```python
from build123d import *

# Parameters (mm, degrees)
CROQUIS1_R              = 2
SALIENTE_EXTRUIR2_DEPTH = 5
CHAFL_N1_SIZE           = 2
CHAFL_N1_SIZE2          = 3.464101615
CROQUIS3_R              = 4
CROQUIS3_R_2            = 1.5
SALIENTE_EXTRUIR3_DEPTH = 5
CROQUIS4_W              = 5
CROQUIS4_H              = 40
SALIENTE_EXTRUIR4_DEPTH = 5
REDONDEO1_R             = 3


with BuildPart() as part:
    # Croquis1 → Saliente-Extruir2 (new body)
    with BuildSketch(Plane(origin=(0, 0, 0), x_dir=(1, 0, 0), z_dir=(0, 1, 0))):
        Polygon((-50, 45), (-50, -45), (50, -45), (50, 45), (15, 45), (15, 30), (-15, 30), (-15, 45), align=None)
        with Locations(Location((-36, -36.5, 0), (0, 0, 270))):
            Circle(CROQUIS1_R, mode=Mode.SUBTRACT)
        with Locations(Location((-36, 36.5, 0), (0, 0, 270))):
            Circle(CROQUIS1_R, mode=Mode.SUBTRACT)
        with Locations(Location((36, 36.5, 0), (0, 0, 270))):
            Circle(CROQUIS1_R, mode=Mode.SUBTRACT)
        with Locations(Location((36, -36.5, 0), (0, 0, 270))):
            Circle(CROQUIS1_R, mode=Mode.SUBTRACT)
    extrude(amount=SALIENTE_EXTRUIR2_DEPTH)

    # Chaflán1
    chafl_n1_edges = [part.edges().sort_by_distance(p)[0] for p in [
        (-36, 5, 34.5),
        (-36, 5, -38.5),
        (36, 5, -38.5),
        (36, 5, 34.5),
    ]]
    chafl_n1_side = [part.faces().sort_by_distance(p)[0] for p in [
        (0, 5, 1.985356127),
    ]]
    chamfer(chafl_n1_edges, length=CHAFL_N1_SIZE, length2=CHAFL_N1_SIZE2, reference=chafl_n1_side[0])

    # Croquis3 → Saliente-Extruir3 (add)
    # profile 1 of 4: a face of its own
    with BuildSketch(Plane(origin=(0, 5, 0), x_dir=(1, 0, 0), z_dir=(0, 1, 0))):
        with Locations(Location((-43.5, -19.5, 0), (0, 0, 270))):
            Circle(CROQUIS3_R)
        with Locations(Location((-43.5, -19.5, 0), (0, 0, 270))):
            Circle(CROQUIS3_R_2, mode=Mode.SUBTRACT)
    # profile 2 of 4: a face of its own
    with BuildSketch(Plane(origin=(0, 5, 0), x_dir=(1, 0, 0), z_dir=(0, 1, 0))):
        with Locations(Location((37, -28, 0), (0, 0, 270))):
            Circle(CROQUIS3_R)
        with Locations(Location((37, -28, 0), (0, 0, 270))):
            Circle(CROQUIS3_R_2, mode=Mode.SUBTRACT)
    # profile 3 of 4: a face of its own
    with BuildSketch(Plane(origin=(0, 5, 0), x_dir=(1, 0, 0), z_dir=(0, 1, 0))):
        with Locations(Location((22, 14, 0), (0, 0, 270))):
            Circle(CROQUIS3_R)
        with Locations(Location((22, 14, 0), (0, 0, 270))):
            Circle(CROQUIS3_R_2, mode=Mode.SUBTRACT)
    # profile 4 of 4: a face of its own
    with BuildSketch(Plane(origin=(0, 5, 0), x_dir=(1, 0, 0), z_dir=(0, 1, 0))):
        with Locations(Location((-21.5, 14, 0), (0, 0, 270))):
            Circle(CROQUIS3_R)
        with Locations(Location((-21.5, 14, 0), (0, 0, 270))):
            Circle(CROQUIS3_R_2, mode=Mode.SUBTRACT)
    extrude(amount=SALIENTE_EXTRUIR3_DEPTH)

    # Croquis4 → Saliente-Extruir4 (add)
    with BuildSketch(Plane(origin=(0, 5, 0), x_dir=(1, 0, 0), z_dir=(0, 1, 0))):
        with Locations((-47.5, 25)):
            Rectangle(CROQUIS4_W, CROQUIS4_H)
        with Locations((47.5, 25)):
            Rectangle(CROQUIS4_W, CROQUIS4_H)
    extrude(amount=SALIENTE_EXTRUIR4_DEPTH)

    # Redondeo1
    redondeo1_edges = [part.edges().sort_by_distance(p)[0] for p in [
        (50, 2.5, 45),
        (-50, 2.5, 45),
        (-50, 5, -45),
        (-15, 2.5, -45),
        (15, 2.5, -45),
        (50, 5, -45),
    ]]
    fillet(redondeo1_edges, radius=REDONDEO1_R)


solid = part.part
```
Check sheet for the modelled part. Datum: model origin and axes. Units: mm. A direction names the side the tool comes from. Give positions to 0.01 mm unless a question says otherwise; leave off trailing zeros. Order: outer loops, then holes, each group sorted by start corner. A loop starts at its lowest first (then second) coordinate and runs counter-clockwise, first axis right, second up. Notation, with made-up numbers: M 29.25,16 L 74.25,16 A14 cw 74.25,33 Z; hole C 69.25,-18 d11. An arc over 180 degrees is marked long. Answer in a Markdown table with one row per item. Add a question column.
Q1. Access from +Z, -Z, +X, -X, +Y, -Y to the whole of each face (thin tool, end or side, straight path). Record for faces 3 (the flat face through (45, 7, -25)), 4 (the flat face through (-45, 7, -25)), 5 (the cylindrical face through (-44.964, 7.465, 19.175)), 6 (the flat face through (47, 7, -5)), 7 (the flat face through (-15, 2, -36)).
Q2. Gauge pin test, flat ends, axial feed: pin 1 Ø5 at (y, z) = (8.5, 33.5) entering from -X; pin 2 Ø10 at (x, z) = (-32.5, 29) entering from +Y; pin 3 Ø1.5 at (x, y) = (46.5, 8.5) entering from +Z; pin 4 Ø4.5 at (x, z) = (-36, -36.5) entering from -Y. Record the tip position at first contact, or that the pin passes through.
Q3. Sectioned sample at A-A, the plane y = 8.25. Count the separate pieces of the cut face and the enclosed holes in it, and give its area (3 significant figures).
Q4. Sectioned sample at B-B, the plane x = -36. Record the boundary of the cut face in (y, z).
Q5. Sectioned sample at C-C, the plane z = -14. Record the boundary of the cut face in (x, y).
Q6. Release check for a two-part mould opening along X. For faces 1 (the cylindrical face through (34.048, 0.757, -36.934)), 2 (the flat face through (-1, 2, 45)) record: released by +X, released by -X, zero draft, split by the parting line, or undercut.
Q7. Sectioned sample at D-D, the plane x = 22. Record the boundary of the cut face in (y, z), and give its area (3 significant figures).
Q8. Thickness scan on L1, parallel to X at y = 0.45, z = -36.5; L2, parallel to X at y = 3.25, z = 35.5; L3, parallel to Y at x = 23.5, z = -5. Record the ranges inside material, lowest first.
Verdict:
| question | item | result |
|---|---|---|
| 1 | face 3 | +Z, -Z, +Y |
| 1 | face 4 | -Z, +Y |
| 1 | face 5 | +Y |
| 1 | face 6 | +Z, +X, -X, +Y |
| 1 | face 7 | -Z, +Y, -Y |
| 2 | pin 1 | x = 34.35 |
| 2 | pin 2 | y = 5 |
| 2 | pin 3 | z = -5 |
| 2 | pin 4 | y = 0 |
| 3 | separate pieces | 6 |
| 3 | enclosed holes | 4 |
| 3 | area | 569 mm² |
| 4 | outline | M 0,-45 L 5,-45 L 5,-40.5 L 1.54,-38.5 L 0,-38.5 Z; M 0,-34.5 L 1.54,-34.5 L 5,-32.5 L 5,32.5 L 1.54,34.5 L 0,34.5 Z; M 0,38.5 L 1.54,38.5 L 5,40.5 L 5,45 L 0,45 Z |
| 5 | outline | M -50,0 L 50,0 L 50,10 L 45,10 L 45,5 L 26,5 L 26,10 L 23.5,10 L 23.5,5 L 20.5,5 L 20.5,10 L 18,10 L 18,5 L -17.5,5 L -17.5,10 L -20,10 L -20,5 L -23,5 L -23,10 L -25.5,10 L -25.5,5 L -45,5 L -45,10 L -50,10 Z |
| 6 | face 1 | undercut |
| 6 | face 2 | zero draft |
| 7 | outline | M 0,-45 L 5,-45 L 5,-18 L 10,-18 L 10,-15.5 L 5,-15.5 L 5,-12.5 L 10,-12.5 L 10,-10 L 5,-10 L 5,45 L 0,45 Z |
| 7 | area | 475 mm² |
| 8 | L1 | -50 to -38, -34 to -15, 15 to 34, 38 to 50 |
| 8 | L2 | -50 to -38.82, -33.18 to 33.18, 38.82 to 50 |
| 8 | L3 | 0 to 5 |
